Design review of the part built by this model. Coordinates are the model's own, in mm. A direction names the side the tool comes from. Coordinates: 2 decimals unless noted, no trailing zeros. Write each loop counter-clockwise with the first axis right and the second up, starting at its lowest first coordinate (ties: lowest second). Pieces come first, ordered by that corner, then holes. Notation, with made-up numbers: (50.25, 26.5) - (54.25, 26.5) arc R16 ccw to (54.25, 54.5) - close; hole circle Ø7 at (19.5, 85). An arc over 180 degrees is marked (long way). Answer as CSV lines item,"result". Start each with the question number.
Q1. We need section D-D (y = 13.75). Write out the cut boundary in (x, z), plus the area to 3 significant figures.
Q2. Mouldability with a two-part tool opening along X and no side actions: class faces 1 (the face through (-16.25, 14, -7)), 2 (the face through (-0.2, 7.3, 0)), 3 (the face through (3.8, 4.25, 0.4)) as pulls with the +X half, pulls with the -X half, needs draft (parallel to the pull), parting line crosses it, or undercut.
Q3. For line 1 along X through (y, z) = (16.25, -2.5); line 2 along Y through (x, z) = (0.9, 1.85); line 3 along Z through (x, y) = (-14.9, 20), list the stretches that pass through material, from the lowest coordinate up. Write a range as [from, to].
Q4. We need section C-C (z = -19.5). Write out the cut boundary in (x, y), plus the area to 3 significant figures.
Q5. Machinability: for faces 4 (the face through (15, 17, -20)), 5 (the face through (-0.227, 4.535, 2.699)), which of the approach directions +Z, -Z, +X, -X, +Y, -Y give a long, thin tool a straight path to every point of the face, cutting with its end or side? Answer none if there is none.
Q6. Clearance check with flat-ended pins moving along their axes: pin 1 (1.8 mm diameter, centred on x = 2.5, y = 6.5, fed in from -Z); pin 2 (4 mm diameter, centred on x = -11, y = 20.5, fed in from -Z) (3 decimals); pin 3 (1.6 mm diameter, centred on x = 15, z = -18, fed in from -Y); pin 4 (3 mm diameter, centred on y = 20, z = -23, fed in from +X). State where each tip first meets the part, or that it passes through.
Q7. We need section B-B (x = 0.9). Write out the cut boundary in (y, z), plus the area to 3 significant figures.
Q8. We need section A-A (z = -23). State how many separate pieces and enclosed holes the cut face has, plus the area to 3 significant figures.
Autodesk Inventor part; units mm, degrees
ref_plane "Work Plane1" through (14.25, 0, 0) normal (1, 0, 0) x (0, 1, 0)
ref_plane "XZ Plane" through (0, 0, 0) normal (0, 1, 0) x (-1, 0, 0)
ref_plane "XY Plane" through (0, 0, 0) normal (0, 0, 1) x (1, 0, 0)
sketch "Sketch1" plane through (0, 0, 0) normal (0, 0, 1) x (1, 0, 0)
  circle A0 centre (-11, 0) radius 1.25 construction
  circle A1 centre (11, 0) radius 1.25 construction
  circle A2 centre (0, -8) radius 12.25 construction
  circle A3 centre (-11, 24) radius 1.5 construction
  circle A4 centre (11, 24) radius 1.5 construction
  line L0 (-14.25, 27.25) -> (14.25, 27.25) construction
  line L1 (14.25, 27.25) -> (14.25, -19.25) construction
  line L2 (14.25, -19.25) -> (-14.25, -19.25) construction
  line L3 (-14.25, -19.25) -> (-14.25, 27.25) construction
  line L4 (-16.25, 10.25) -> (16.25, 10.25)
  line L5 (16.25, 10.25) -> (16.25, 4.25)
  line L6 (16.25, 4.25) -> (-16.25, 4.25)
  line L7 (-16.25, 4.25) -> (-16.25, 10.25)
  circle A5 centre (0.9, 7.25) radius 0.9
  line L8 (0, 4.25) -> (0, 10.25) construction
  circle A6 centre (0, -8) radius 9.5 construction
  point P0 (0, 0)
  point P1 (0, 27.25)
  point P2 (16.25, 7.25)
  dimension "d0" = 2.5
  dimension "d1" = 2.5
  dimension "d2" = 22
  dimension "d3" = 11
  dimension "d4" = 8
  dimension "d5" = 24.5
  dimension "d6" = 3
  dimension "d7" = 3
  dimension "d8" = 24
  dimension "d9" = 28.5
  dimension "d10" = 3.25
  dimension "d11" = 46.5
  dimension "d12" = 2
  dimension "d13" = 6
  dimension "d14" = 1.8
  dimension "d15" = 19
extrude "Extrusion1" add sketch "Sketch1" along normal blind 3
ref_plane "Work Plane1" through (14.25, 0, 0) normal (1, 0, 0) x (0, 1, 0)
sketch "Sketch2" plane through (14.25, 0, 0) normal (1, 0, 0) x (0, 1, 0)
  line L0 (4.25, 0) -> (10.25, 0)
  circle A0 centre (20, -11) radius 1.25
  circle A1 centre (20, -23) radius 1.25
  line L1 (17, -26) -> (23, -26)
  line L2 (23, -26) -> (23, -6)
  line L3 (23, -6) -> (17, -6) construction
  line L4 (17, -6) -> (17, -26)
  line L5 (4.25, 0) -> (23, 0)
  line L6 (23, 0) -> (23, -6)
  line L7 (23, -6) -> (4.25, -6) construction
  line L8 (4.25, -6) -> (4.25, 0)
  line L9 (4.25, -6) -> (17, -6)
  point P0 (0, 0)
  point P1 (27.25, 0)
  point P2 (27.25, 0)
  point P3 (27.25, 0)
  point P4 (20, -26)
  dimension "d19" = 7.25
  dimension "d20" = 11
  dimension "d21" = 12
  dimension "d22" = 2.5
  dimension "d23" = 2.5
  dimension "d24" = 3
  dimension "d25" = 3
  dimension "d26" = 6
extrude "Extrusion2" add sketch "Sketch2" along normal up to surface (2 mm away)
fillet "Fillet1" radius 10 2 edges at (15.25, 17, -6) (15.25, 23, 0)
fillet "Fillet1" radius 2 4 edges at (15.25, 4.25, -6) (15.25, 17, -26) (15.25, 23, -26) (15.25, 10.25, 0)
mirror "Mirror1" about plane through (0, 0, 0) normal (1, 0, 0) of "Extrusion2", "Fillet1"
fillet "Fillet2" radius 1 2 edges at (0, 10.25, 3) (0, 4.25, 3)
sketch "Sketch3" plane through (-16.25, 19, -26) normal (-1, 0, 0) x (0, 0, 1)
  arc A0 (2, 4) -> (0, 2) centre (2, 2) ccw construction
  line L0 (2, 4) -> (16, 4) construction
  arc A1 (26, -6) -> (16, 4) centre (16, -6) ccw construction
  line L1 (26, -6) -> (26, -6.75) construction
  arc A2 (26, -6.75) -> (28, -8.75) centre (28, -6.75) ccw construction
  arc A3 (29, -9.75) -> (28, -8.75) centre (28, -9.75) ccw construction
  line L2 (29, -9.75) -> (29, -13.75) construction
  arc A4 (28, -14.75) -> (29, -13.75) centre (28, -13.75) ccw construction
  line L3 (28, -14.75) -> (22, -14.75) construction
  arc A5 (20, -12.75) -> (22, -14.75) centre (22, -12.75) ccw construction
  line L4 (20, -12.75) -> (20, -12) construction
  arc A6 (20, -12) -> (10, -2) centre (10, -12) ccw construction
  line L5 (10, -2) -> (2, -2) construction
  arc A7 (0, 0) -> (2, -2) centre (2, 0) ccw construction
  line L6 (0, 0) -> (0, 2) construction
  circle A8 centre (15, 1) radius 1.25
  circle A9 centre (3, 1) radius 1.25 construction
  circle A10 centre (3, 1) radius 1.25
  circle A11 centre (3, 1) radius 2
  circle A12 centre (15, 1) radius 2
  point P0 (26, -19)
  dimension "d32" = 4
  dimension "d33" = 4
extrude "Extrusion3" add sketch "Sketch3" along normal blind 1
fillet "Fillet3" radius 1 2 edges at (-16.25, 20, -25) (-16.25, 20, -13)
mirror "Mirror2" about plane through (0, 0, 0) normal (1, 0, 0) of "Extrusion3", "Fillet3"
equation "\"d7\" = d6"
equation "\"d23\" = d22"
equation "\"d25\" = d24"
equation "\"d33\" = d32"
properties part number "Tendon_Center"
Results list:
1,outline,"(-16.25, -8.62) - (-14.25, -8.62) - (-14.25, -0.03) - (-16.25, -0.03) - close; (14.25, -8.62) - (16.25, -8.62) - (16.25, -0.03) - (14.25, -0.03) - close"
1,area,"34.4 mm2"
2,face 1,"pulls with the -X half"
2,face 2,"undercut"
2,face 3,"needs draft"
3,line 1,"x = [-16.25, -14.25], [14.25, 16.25]"
3,line 2,"y = [4.25, 6.35], [8.15, 10.25]"
3,line 3,"z = [-26, -24.25], [-21.75, -12.25], [-9.75, -2.86]"
4,outline,"(-16.25, 17) - (-14.25, 17) - (-14.25, 23) - (-16.25, 23) - close; (14.25, 17) - (16.25, 17) - (16.25, 23) - (14.25, 23) - close"
4,area,"24.0 mm2"
5,face 4,"-Z, +X, -X, -Y"
5,face 5,"+Z, +X, -X, -Y"
6,pin 1,"stops at z = 0"
6,pin 2,"passes through"
6,pin 3,"stops at y = 17"
6,pin 4,"stops at x = 17.25"
7,outline,"(4.25, 0) - (6.35, 0) - (6.35, 3) - (5.25, 3) arc R1 ccw to (4.25, 2) - close; (8.15, 0) - (10.25, 0) - (10.25, 2) arc R1 ccw to (9.25, 3) - (8.15, 3) - close"
7,area,"12.2 mm2"
8,separate pieces,"4"
8,enclosed holes,"0"
8,area,"17.9 mm2"
